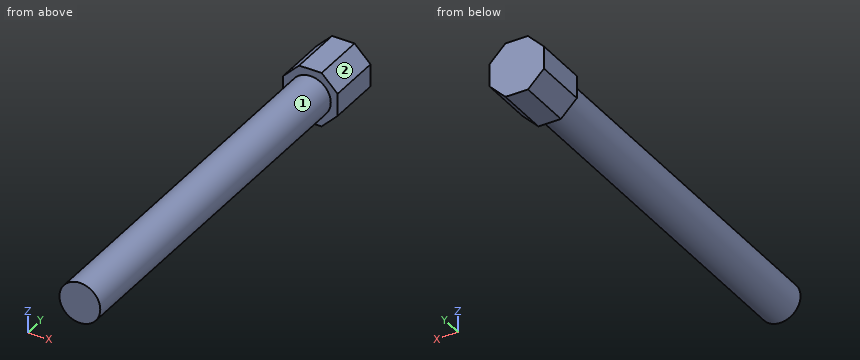
from build123d import *

# Parameters (mm, degrees)
F0_R     = 4.7625
F1_DEPTH = 101.6
F3_DEPTH = 12.7


with BuildPart() as f1:
    # F0 (on Front) → F1 (new body)
    with BuildSketch(Plane.XZ):
        Circle(F0_R)
    extrude(amount=F1_DEPTH)

    # F2 (on Front) → F3 (join)
    with BuildSketch(Plane.XZ):
        Polygon((-2.630256, -6.35), (2.630256, -6.35), (6.35, -2.630256), (6.35, 2.630256), (2.630256, 6.35), (-2.630256, 6.35), (-6.35, 2.630256), (-6.35, -2.630256), align=None)
    extrude(amount=F3_DEPTH)


solid = f1.part
Input: part model. Units: mm. Frame: model coordinates. Face numbers are marked on the shaded views. A direction names the side the tool comes from. Round coordinates to 2 decimals unless told otherwise and drop trailing zeros. Write each loop counter-clockwise with the first axis right and the second up, starting at its lowest first coordinate (ties: lowest second). Pieces come first, ordered by that corner, then holes.
1) Cut plane C-C (y = -52.5). Return the cut outline in (x, z) (1 decimal).
2) Cut plane B-B (z = 0). Return the cut outline in (x, y).
3) Reachability of the marked faces 1 and 2 from +Z, -Z, +X, -X, +Y, -Y: full face, straight path, thin tool, end or side. Return the list, or none.
4) Ray query, L1, parallel to Y at x = -4.25, z = 4.25; L2, parallel to Z at x = 0, y = -18.5; L3, parallel to Z at x = 2, y = -50. Return the intervals inside material, ascending.
5) Contact query for flat-ended pins moving along their axis: P1, Ø1.5, axis at x = -1.5, y = -33, coming from the -Z side; P2, Ø2, axis at y = -83, z = -2.5, coming from the +X side; P3, Ø6, axis at x = 5, y = -60, coming from the -Z side. Output: stop coordinate, or through.
6) Cut plane A-A (x = 0). Return the cut outline in (y, z).
Geometry says:
1. outline: circle Ø9.5 at (0, 0)
2. outline: (-6.35, -12.7) - (-4.76, -12.7) - (-4.76, -101.6) - (4.76, -101.6) - (4.76, -12.7) - (6.35, -12.7) - (6.35, 0) - (-6.35, 0) - close
3. face 1: -Y
3. face 2: +Z, +X, +Y, -Y
4. L1: y = -12.7 to 0
4. L2: z = -4.76 to 4.76
4. L3: z = -4.32 to 4.32
5. P1: stops at z = -4.7
5. P2: stops at x = 4.52
5. P3: stops at z = -4.32
6. outline: (-101.6, -4.76) - (-12.7, -4.76) - (-12.7, -6.35) - (0, -6.35) - (0, 6.35) - (-12.7, 6.35) - (-12.7, 4.76) - (-101.6, 4.76) - close
